from build123d import *

# Parameters (mm, degrees)
SKETCH1_W             = 15.875
SKETCH1_H             = 15.875
BOSS_EXTRUDE1_DEPTH   = 9.525
F_5_40_TAPPED_HOLE1_D = 2.5781
SKETCH4_R             = 3.937
BOSS_EXTRUDE2_DEPTH   = 1.143
SKETCH10_R            = 1.9685
BOSS_EXTRUDE4_DEPTH   = 4.953
F_4_40_TAPPED_HOLE1_D = 2.2606
SKETCH9_OUTSIDE_W     = 23.345
SKETCH9_OUTSIDE_H     = 23.345
SKETCH9_OUTSIDE_R     = 3.175
CUT_EXTRUDE3_DEPTH    = 3.175
SKETCH11_OUTSIDE_W    = 23.345
SKETCH11_OUTSIDE_H    = 23.345
CUT_EXTRUDE4_DEPTH    = 15.721869362
CHAMFER1_SIZE         = 0.254
CHAMFER3_SIZE         = 0.508
CHAMFER4_SIZE         = 0.127


with BuildPart() as part:
    # Sketch1 → Boss-Extrude1 (new body)
    with BuildSketch(Plane(origin=(0, 0, 0), x_dir=(1, 0, 0), z_dir=(0, 1, 0))):
        Rectangle(SKETCH1_W, SKETCH1_H)
    extrude(amount=BOSS_EXTRUDE1_DEPTH)

    # #5-40 Tapped Hole1 (through all)
    with Locations(Plane(origin=(0, 0, 0), x_dir=(-1, 0, 0), z_dir=(0, -1, 0))):
        with Locations((-5.8039, -5.8039), (-5.8039, 5.8039), (5.8039, 5.8039), (5.8039, -5.8039)):
            Hole(F_5_40_TAPPED_HOLE1_D / 2)

    # Sketch4 → Boss-Extrude2 (add)
    with BuildSketch(Plane.XZ):
        with Locations(Location((0, 0, 0), (0, 0, 90))):
            Circle(SKETCH4_R)
    extrude(amount=BOSS_EXTRUDE2_DEPTH)

    # Sketch10 → Boss-Extrude4 (add)
    with BuildSketch(Plane.XZ.offset(1.143)):
        with Locations(Location((0, 0, 0), (0, 0, 90))):
            Circle(SKETCH10_R)
    extrude(amount=BOSS_EXTRUDE4_DEPTH)

    # #4-40 Tapped Hole1 (through all)
    with Locations(Plane(origin=(0, -6.096, 0), x_dir=(-1, 0, 0), z_dir=(0, -1, 0))):
        with Locations((0, 0)):
            Hole(F_4_40_TAPPED_HOLE1_D / 2)

    # Sketch9 outside → Cut-Extrude3 (cut)
    with BuildSketch(Plane(origin=(0, 9.525, 0), x_dir=(1, 0, 0), z_dir=(0, 1, 0))):
        with Locations((-0.0005, -0.0005)):
            Rectangle(SKETCH9_OUTSIDE_W, SKETCH9_OUTSIDE_H)
        with Locations(Location((0, 0, 0), (0, 0, 270))):
            Circle(SKETCH9_OUTSIDE_R, mode=Mode.SUBTRACT)
    extrude(amount=-CUT_EXTRUDE3_DEPTH, mode=Mode.SUBTRACT)

    # Sketch11 outside → Cut-Extrude4 (cut, through all)
    with BuildSketch(Plane.XZ):
        with Locations((-0.0005, 0.0005)):
            Rectangle(SKETCH11_OUTSIDE_W, SKETCH11_OUTSIDE_H)
        with BuildLine():
            Line((-5.8039, 7.9375), (5.8039, 7.9375))
            ThreePointArc((5.8039, 7.9375), (7.312583028, 7.312583028), (7.9375, 5.8039))
            Line((7.9375, 5.8039), (7.9375, -5.8039))
            ThreePointArc((7.9375, -5.8039), (7.312583028, -7.312583028), (5.8039, -7.9375))
            Line((5.8039, -7.9375), (-5.8039, -7.9375))
            ThreePointArc((-5.8039, -7.9375), (-7.312583028, -7.312583028), (-7.9375, -5.8039))
            Line((-7.9375, -5.8039), (-7.9375, 5.8039))
            ThreePointArc((-7.9375, 5.8039), (-7.312583028, 7.312583028), (-5.8039, 7.9375))
        make_face(mode=Mode.SUBTRACT)
    extrude(amount=-CUT_EXTRUDE4_DEPTH, mode=Mode.SUBTRACT)

    # Chamfer1
    chamfer1_edges = [part.edges().sort_by_distance(p)[0] for p in [
        (0, -1.143, -3.937),
        (0, -6.096, -1.9685),
    ]]
    chamfer(chamfer1_edges, length=CHAMFER1_SIZE)

    # Chamfer3
    chamfer3_edges = [part.edges().sort_by_distance(p)[0] for p in [
        (0, 9.525, -3.175),
        (7.9375, 6.35, 0),
        (0, 6.35, -7.9375),
        (-7.9375, 6.35, 0),
        (0, 6.35, 7.9375),
        (-7.312583028, 6.35, -7.312583028),
        (7.312583028, 6.35, -7.312583028),
        (7.312583028, 6.35, 7.312583028),
        (-7.312583028, 6.35, 7.312583028),
    ]]
    chamfer(chamfer3_edges, length=CHAMFER3_SIZE)

    # Chamfer4
    chamfer4_edges = [part.edges().sort_by_distance(p)[0] for p in [
        (-7.312583028, 0, 7.312583028),
        (7.312583028, 0, 7.312583028),
        (7.312583028, 0, -7.312583028),
        (-7.312583028, 0, -7.312583028),
        (7.9375, 0, 0),
        (0, 0, 7.9375),
        (-7.9375, 0, 0),
        (0, 0, -7.9375),
    ]]
    chamfer(chamfer4_edges, length=CHAMFER4_SIZE)


solid = part.part
The listing builds one solid part. Answer for the finished solid, in the listing's coordinates (mm). A direction names the side the tool comes from. Give positions to 0.01 mm unless a question says otherwise; leave off trailing zeros. Order: outer loops, then holes, each group sorted by start corner. A loop starts at its lowest first (then second) coordinate and runs counter-clockwise, first axis right, second up. Notation, with made-up numbers: (-18.5, 71.25) - (37.5, 71.25) arc R36 cw to (37.5, 105.25) - close; hole circle Ø4 at (84.25, -31.5). An arc over 180 degrees is marked (long way). One line per item, written item: value. Start each with the question number.
1) A tool of negligible diameter and unlimited length cuts with its end or side. For faces 5 (the face through (0, 3, -7.938)), 6 (the face through (-1.93, 7.7, -2.52)), 7 (the face through (3.843, -0.438, -0.853)), from which of +Z, -Z, +X, -X, +Y, -Y can it reach the whole face along a straight path? Write none if from no direction.
2) The mould has two halves that part along X. Classify faces 1 (the face through (7.329, 2.944, -7.296)), 2 (the face through (4.78, 3.22, 6.59)), 3 (the face through (-2, 0, -4)), 4 (the face through (1.92, -3.46, -0.43)): released by +X, released by -X, zero draft, split by the parting line, or undercut.
3) Given pin 1 Ø2 at (x, z) = (-5.8, 5.8) entering from -Y; pin 2 Ø4 at (x, z) = (5.8, 5.8) entering from -Y; pin 3 Ø2 at (x, z) = (-4, -1) entering from +Y; pin 4 Ø3.5 at (x, z) = (5.8, -5.8) entering from +Y, each flat-ended and moving along its own axis, determine where each tip first touches the part or whether it passes through.
4) A cutting plane is placed at D-D on x = 5.5. Give the vertices of the cut face in (y, z).
5) Find the intervals of material crossed by L1, parallel to Y at x = 4.75, z = 7; L2, parallel to Y at x = -1.25, z = -2.25 (3 decimals); L3, parallel to X at y = 7, z = 0.75, in increasing order.
6) A cutting plane is placed at C-C on y = 1. Give the vertices of the cut face in (x, z), then the cut area to 3 significant figures.
Answer sheet:
1. face 5: -Z, +X, -X, +Y, -Y
1. face 6: +Y
1. face 7: -Y
2. face 1: released by +X
2. face 2: undercut
2. face 3: zero draft
2. face 4: split by the parting line
3. pin 1: passes through
3. pin 2: stops at y = 0
3. pin 3: stops at y = 9.07
3. pin 4: stops at y = 6.35
4. outline: (0, -7.81) - (0.13, -7.94) - (5.84, -7.94) - (6.35, -7.43) - (6.35, -7.06) - (0, -7.06) - close; (0, -4.55) - (6.35, -4.55) - (6.35, 4.55) - (0, 4.55) - close; (0, 7.06) - (6.35, 7.06) - (6.35, 7.43) - (5.84, 7.94) - (0.13, 7.94) - (0, 7.81) - close
5. L1: y = 0 to 6.35
5. L2: y = -1.143 to 9.525
5. L3: x = -3.09 to -0.85, 0.85 to 3.09
6. outline: (-7.94, -5.8) arc R2.13 ccw to (-5.8, -7.94) - (5.8, -7.94) arc R2.13 ccw to (7.94, -5.8) - (7.94, 5.8) arc R2.13 ccw to (5.8, 7.94) - (-5.8, 7.94) arc R2.13 ccw to (-7.94, 5.8) - close; hole circle Ø2.58 at (-5.8, -5.8); hole circle Ø2.58 at (-5.8, 5.8); hole circle Ø2.26 at (0, 0); hole circle Ø2.58 at (5.8, -5.8); hole circle Ø2.58 at (5.8, 5.8)
6. area: 223 mm2
